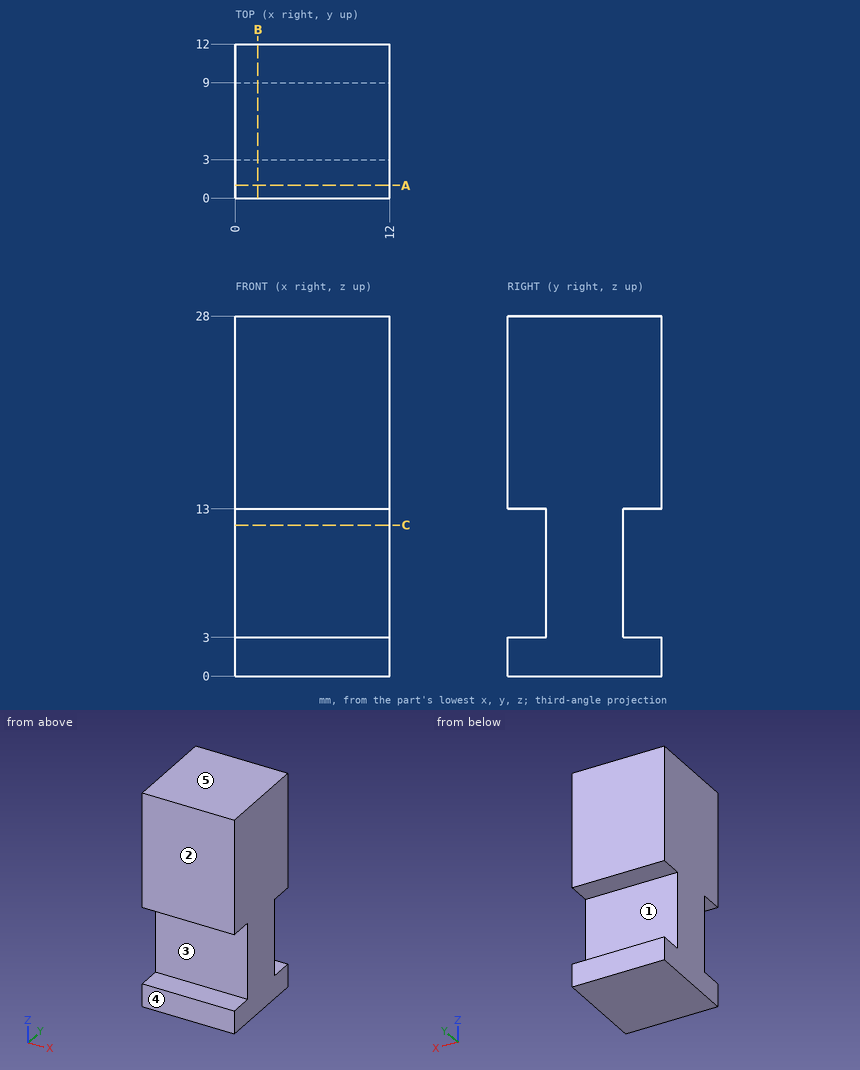
Geometry check sheet. Reference: drawing and pictorial views, mm from the part's lowest x, y, z. A direction names the side the tool comes from. Give positions to 0.01 mm unless a question says otherwise; leave off trailing zeros. Write each loop counter-clockwise with the first axis right and the second up, starting at its lowest first coordinate (ties: lowest second). Pieces come first, ordered by that corner, then holes. Notation, with made-up numbers: M 46,30.5 L 75,30.5 A21 ccw 75,38.5 Z; hole C -7,83.25 d6. An arc over 180 degrees is marked long. Put each result on its own line as item: value. Start each with the question number.
1. Go/stop test with flat-tipped pins: pin 1 Ø3 at (y, z) = (2.5, 7.5) entering from +X; pin 2 Ø1 at (x, z) = (6.5, 7) entering from +Y. Record where each tip stops, or that it passes through.
2. Section check C-C (z = 11.75). Record the cut outline in (x, y).
3. Draft check along Z on the marked faces 3, 4 and 5. Enter one of: +Z half, -Z half, draft (parallel to the pull), parting line (faces both ways), or undercut.
4. Scan lines: line 1 along Z through (x, y) = (4, 2); line 2 along Y through (x, z) = (2.25, 11.75). Record each from-to range of solid material in increasing order. Write a range as [from, to].
5. Section check A-A (y = 1). Record the cut outline in (x, z), and give its area (3 significant figures).
6. Set-up check for the marked faces 1 and 2: record each of +Z, -Z, +X, -X, +Y, -Y from which the full face is reachable in a straight line by a thin tool's end or side.
7. Section check B-B (x = 1.75). Record the cut outline in (y, z).
Answer list:
1. pin 1: x = 12
1. pin 2: y = 9
2. outline: M 0,3 L 12,3 L 12,9 L 0,9 Z
3. face 3: undercut
3. face 4: draft
3. face 5: +Z half
4. line 1: [0, 3], [13, 28]
4. line 2: [3, 9]
5. outline: M 0,0 L 12,0 L 12,3 L 0,3 Z; M 0,13 L 12,13 L 12,28 L 0,28 Z
5. area: 216 mm2
6. face 1: +X, -X, +Y
6. face 2: +Z, -Z, +X, -X, -Y
7. outline: M 0,0 L 12,0 L 12,3 L 9,3 L 9,13 L 12,13 L 12,28 L 0,28 L 0,13 L 3,13 L 3,3 L 0,3 Z
